Can you work these out from the model? Positions are in its coordinate system, mm. A direction names the side the tool comes from. Give positions to 0.01 mm unless a question says otherwise; leave off trailing zeros. Order: outer loops, then holes, each group sorted by start corner. A loop starts at its lowest first (then second) coordinate and runs counter-clockwise, first axis right, second up. Notation, with made-up numbers: (68.5, 69) - (111.5, 69) arc R26 ccw to (111.5, 93) - close; hole circle Ø11 at (72.25, 19). An arc over 180 degrees is marked (long way). Use one line per item in the form item = value. Start each with the question number.
1) Please list where these lines run through material, in increasing order: probe 1 along X at (y, z) = (7.4, 0); probe 2 along X at (y, z) = (5.35, 0); probe 3 along X at (y, z) = (4.65, 0).
2) Which directions (+Z, -Z, +X, -X, +Y, -Y) give clear straight access to the entire face, cutting with the end or side of a thin tool? Please do faces 5 (the flat face through (0, -7.5, 0)), 6 (the flat face through (0, 4, 0)), 7 (the flat face through (-5, 7.5, 0)), 8 (the flat face through (85, 0, 0)).
3) For pin 1 (10.5 mm diameter, centred on x = 40, z = 1.5, fed in from -Y); pin 2 (3 mm diameter, centred on x = 0, z = 0, fed in from +Y); pin 3 (5.5 mm diameter, centred on x = 1, z = -1, fed in from +Y), each with a flat end and sliding along its axis, tell me the tip position at first contact or that it passes through.
4) Suppose I cut it at B-B, the plane z = 0. Write out the boundary of the cut face in (x, y), and give its area (3 significant figures).
5) Suppose I cut it at C-C, the plane y = -1.25. Write out the boundary of the cut face in (x, z).
6) We'd pull the mould along Z, two halves only. Please class faces 1 (the cylindrical face through (-21.965, 0.105, -4.878)), 2 (the flat face through (51, 6.466, 0)), 3 (the cylindrical face through (-1, 6, 0)), 4 (the cylindrical face through (-2.44, 7.25, -0.54)): released by +Z, released by -Z, zero draft, split by the parting line, or undercut.
7) Suppose I cut it at A-A, the plane x = 0. Write out the boundary of the cut face in (y, z).
8) Suppose I cut it at D-D, the plane x = 49. Write out the boundary of the cut face in (y, z), and give its area (3 significant figures).
```python
from build123d import *

# Parameters (mm, degrees)
SKETCH_1_R           = 22.5
EXTRUDE_1_DEPTH      = 7.5
SKETCH_3_R           = 7.5
EXTRUDE_2_DEPTH      = 7.5
SKETCH_4_W           = 23.480524837
SKETCH_4_H           = 9.129078989
CUT_EXTRUDE_2_DEPTH  = 97.083765538
EXTRUDE_3_REACH      = 113.978
EXTRUDE_3_END_RADIUS = 22.5
SKETCH_5_W           = 10
SKETCH_5_H           = 1.436694835
SKETCH_6_R           = 2.5
CUT_EXTRUDE_3_DEPTH  = 0.5
SKETCH_7_R           = 1
CUT_EXTRUDE_4_DEPTH  = 3
FILLET_1_R           = 0.3


with BuildPart() as part:
    # Sketch 1 → Extrude 1 (new, symmetric)
    with BuildSketch(Plane(origin=(0, 0, 0), x_dir=(1, 0, 0), z_dir=(0, 1, 0))):
        with Locations(Location((0, 0, 0), (0, 0, 270))):
            Circle(SKETCH_1_R)
    extrude(amount=EXTRUDE_1_DEPTH, both=True)



with BuildPart() as body_2:
    # Sketch 3 → Extrude 2 (new, symmetric)
    with BuildSketch(Plane(origin=(0, 7.5, 0), x_dir=(1, 0, 0), z_dir=(0, 1, 0))):
        with Locations(Location((84.7, 0, 0), (0, 0, 270))):
            Circle(SKETCH_3_R)
    extrude(amount=EXTRUDE_2_DEPTH, both=True)

    # Sketch 4 → Cut-Extrude 2 (cut, through all)
    with BuildSketch(Plane(origin=(0, 0, 0), x_dir=(0, 0, -1), z_dir=(1, 0, 0))):
        with Locations((0.499792143, 13.617320583)):
            Rectangle(SKETCH_4_W, SKETCH_4_H)
    extrude(amount=CUT_EXTRUDE_2_DEPTH, mode=Mode.SUBTRACT)


with BuildPart() as part_1:
    add(part.part)

    add(body_2.part)  # Extrude 3 merges body 2
    # Extrude 3: up to this cylinder (the profile starts outside it)
    extrude_3_end = Plane(origin=(0, 5.748089, 0), z_dir=(0, -1, 0)) * Cylinder(EXTRUDE_3_END_RADIUS, 273.956, mode=Mode.PRIVATE)
    # Sketch 5 → Extrude 3 (add, up to the surface)
    with BuildSketch(Plane(origin=(86.82, 0, 0), x_dir=(0, 0, -1), z_dir=(1, 0, 0)), mode=Mode.PRIVATE) as extrude_3_sk1:
        with Locations((0, 5.748089048)):
            Rectangle(SKETCH_5_W, SKETCH_5_H)
    extrude_3_tool1 = extrude(extrude_3_sk1.sketch, amount=-EXTRUDE_3_REACH, mode=Mode.PRIVATE) - extrude_3_end
    add(extrude_3_tool1.solids().sort_by_distance((86.82, 5.748089, 0))[0])

    # Sketch 6 → Cut-Extrude 3 (cut)
    with BuildSketch(Plane(origin=(0, 7.5, 0), x_dir=(1, 0, 0), z_dir=(0, 1, 0))):
        with Locations(Location((0, 0, 0), (0, 0, 270))):
            Circle(SKETCH_6_R)
    extrude(amount=-CUT_EXTRUDE_3_DEPTH, mode=Mode.SUBTRACT)

    # Sketch 7 → Cut-Extrude 4 (cut)
    with BuildSketch(Plane(origin=(0, 7, 0), x_dir=(1, 0, 0), z_dir=(0, 1, 0))):
        with Locations(Location((0, 0, 0), (0, 0, 270))):
            Circle(SKETCH_7_R)
    extrude(amount=-CUT_EXTRUDE_4_DEPTH, mode=Mode.SUBTRACT)

    # Fillet 1
    fillet_1_edges = [part_1.edges().sort_by_distance(p)[0] for p in [
        (50.523620512, 6.466436465, 5),
        (50.523620512, 5.02974163, -5),
        (50.523620512, 5.02974163, 5),
        (50.523620512, 6.466436465, -5),
    ]]
    fillet(fillet_1_edges, radius=FILLET_1_R)


solid = part_1.part
```
Result sheet:
q1.probe_1 = -22.5 to -2.5, 2.5 to 22.5, 77.2 to 92.2
q1.probe_2 = -22.5 to -1, 1 to 92.2
q1.probe_3 = -22.5 to -1, 1 to 22.5, 77.2 to 92.2
q2.face_5 = +Z, -Z, +X, -X, -Y
q2.face_6 = +Y
q2.face_7 = +Z, -Z, -X, +Y
q2.face_8 = +Z, -Z, +X, -Y
q3.pin_1 = 5.03
q3.pin_2 = 7
q3.pin_3 = 7.5
q4.outline = (-22.5, -7.5) - (22.5, -7.5) - (22.5, 5.03) - (77.2, 5.03) - (77.2, 0) - (92.2, 0) - (92.2, 9.05) - (77.2, 9.05) - (77.2, 6.47) - (22.5, 6.47) - (22.5, 7.5) - (2.5, 7.5) - (2.5, 7) - (1, 7) - (1, 4) - (-1, 4) - (-1, 7) - (-2.5, 7) - (-2.5, 7.5) - (-22.5, 7.5) - close
q4.area = 881 mm²
q5.outline = circle Ø45 at (0, 0)
q6.face_1 = split by the parting line
q6.face_2 = zero draft
q6.face_3 = undercut
q6.face_4 = undercut
q7.outline = (-7.5, -22.5) - (7.5, -22.5) - (7.5, -2.5) - (7, -2.5) - (7, -1) - (4, -1) - (4, 1) - (7, 1) - (7, 2.5) - (7.5, 2.5) - (7.5, 22.5) - (-7.5, 22.5) - close
q8.outline = (5.03, -4.7) arc R0.3 ccw to (5.33, -5) - (6.17, -5) arc R0.3 ccw to (6.47, -4.7) - (6.47, 4.7) arc R0.3 ccw to (6.17, 5) - (5.33, 5) arc R0.3 ccw to (5.03, 4.7) - close
q8.area = 14.3 mm²
